Read the model definition and answer for the solid it produces. Units are mm, in the model's axes. A direction names the side the tool comes from. Round coordinates to 2 decimals unless told otherwise and drop trailing zeros. Order: outer loops, then holes, each group sorted by start corner. A loop starts at its lowest first (then second) coordinate and runs counter-clockwise, first axis right, second up. Notation, with made-up numbers: (70.25, 54.25) -> (78.25, 54.25) arc R9 cw to (78.25, 66.25) -> close; hole circle Ø2 at (89, 15). An arc over 180 degrees is marked (long way). One line per item, written item: value. Start each with the question number.
1. Section A-A (z = -1.5) is taken. Give the vertices of the cut face in (x, y).
2. Consider line 1 (Y direction, x = 12, z = 1.05); line 2 (Y direction, x = -12, z = 2.6); line 3 (Y direction, x = 5.5, z = 9.5). Determine where each line is inside the solid, lowest interval first.
3. Section B-B (x = 0) is taken. Give the vertices of the cut face in (y, z) (3 decimals).
4. Section D-D (z = 6.5) is taken. Give the vertices of the cut face in (x, y), then the cut area to 3 significant figures.
5. Section C-C (y = 70.5) is taken. Give the vertices of the cut face in (x, z), then the cut area to 3 significant figures.
6. The mould has two halves that part along Y. Classify faces 4 (the face through (-0.275, 132.886, 12.497)), 5 (the face through (-15.5, 77, 8)), 6 (the face through (0, 2, 9)), 7 (the face through (-12, 147, 3.5)): released by +Y, released by -Y, zero draft, split by the parting line, or undercut.
7. For faces 1 (the face through (0, 63, 8)), 2 (the face through (11.1, 148.5, -1.7)), 3 (the face through (0, 77, 15.5)), determine the directions among +Z, -Z, +X, -X, +Y, -Y from which every point of the face is accessible in a straight line to the end or side of a thin tool.
8. Flat-ended cylindrical pins translate along their axes: pin 1 Ø4 at (x, y) = (9.5, 83.5) entering from -Z; pin 2 Ø1 at (x, y) = (-12.5, 147) entering from -Z. Find the tip coordinate at first contact, or state that the pin passes through.
from build123d import *

# Parameters (mm, degrees)
SKETCH1_R            = 12.5
BOSS_EXTRUDE1_DEPTH  = 150.5
BOSS_EXTRUDE2_DEPTH  = 148.5
SKETCH8_R            = 12.5
CUT_EXTRUDE2_DEPTH   = 152.706130397
BOSS_EXTRUDE7_DEPTH  = 8
BOSS_EXTRUDE8_START  = -121
BOSS_EXTRUDE8_DEPTH  = 121
BOSS_EXTRUDE9_DEPTH  = 148.5
SKETCH13_R           = 1.75
CUT_EXTRUDE3_DEPTH   = 3.5
SKETCH14_R           = 1.75
BOSS_EXTRUDE10_DEPTH = 3.4
SKETCH15_R           = 1.75
CUT_EXTRUDE4_DEPTH   = 3.5
SKETCH16_R           = 1.75
BOSS_EXTRUDE11_DEPTH = 3.4


with BuildPart() as part:
    # Sketch1 → Boss-Extrude1 (new body)
    with BuildSketch(Plane(origin=(0, 0, 0), x_dir=(1, 0, 0), z_dir=(0, 1, 0))):
        with Locations(Location((0, 0, 0), (0, 0, 270))):
            Circle(SKETCH1_R)
    extrude(amount=BOSS_EXTRUDE1_DEPTH)

    # Sketch2 → Boss-Extrude2 (add)
    with BuildSketch(Plane(origin=(0, 150.5, 0), x_dir=(1, 0, 0), z_dir=(0, 1, 0))):
        with BuildLine():
            Line((-13.5, 0), (13.5, 0))
            ThreePointArc((13.5, 0), (0, -13.5), (-13.5, 0))
        make_face()
    extrude(amount=-BOSS_EXTRUDE2_DEPTH)

    # Sketch8 → Cut-Extrude2 (cut, through all)
    with BuildSketch(Plane(origin=(0, 150.5, 0), x_dir=(1, 0, 0), z_dir=(0, 1, 0))):
        Circle(SKETCH8_R)
    extrude(amount=-CUT_EXTRUDE2_DEPTH, mode=Mode.SUBTRACT)

    # Sketch9 → Boss-Extrude7 (add)
    with BuildSketch(Plane(origin=(0, 150.5, 0), x_dir=(1, 0, 0), z_dir=(0, 1, 0))):
        with BuildLine():
            Line((12.5, 0), (1.875, 0))
            ThreePointArc((1.875, 0), (0, -1.875), (-1.875, 0))
            Line((-1.875, 0), (-12.5, 0))
            ThreePointArc((-12.5, 0), (0, -12.5), (12.5, 0))
        make_face()
    extrude(amount=-BOSS_EXTRUDE7_DEPTH)

    # Sketch11 → Boss-Extrude8 (add)
    with BuildSketch(Plane.XZ.offset(-2).offset(BOSS_EXTRUDE8_START)):
        with BuildLine():
            Line((-12.5, 0), (-8, 0))
            ThreePointArc((-8, 0), (0, 8), (8, 0))
            Line((8, 0), (12.5, 0))
            ThreePointArc((12.5, 0), (0, 12.5), (-12.5, 0))
        make_face()
    extrude(amount=BOSS_EXTRUDE8_DEPTH)

    # Sketch12 → Boss-Extrude9 (add)
    with BuildSketch(Plane(origin=(0, 150.5, 0), x_dir=(1, 0, 0), z_dir=(0, 1, 0))):
        with BuildLine():
            Line((-13.5, 0), (-15.5, 0))
            Line((-15.5, 0), (-15.5, -15.5))
            Line((-15.5, -15.5), (15.5, -15.5))
            Line((15.5, -15.5), (15.5, 0))
            Line((15.5, 0), (13.5, 0))
            ThreePointArc((13.5, 0), (0, -13.5), (-13.5, 0))
        make_face()
    extrude(amount=-BOSS_EXTRUDE9_DEPTH)

    # Sketch13 → Cut-Extrude3 (cut)
    with BuildSketch(Plane(origin=(0, 0, 0), x_dir=(-1, 0, 0), z_dir=(0, 0, -1))):
        with Locations((12, 147)):
            Circle(SKETCH13_R)
    extrude(amount=-CUT_EXTRUDE3_DEPTH, mode=Mode.SUBTRACT)

    # Sketch14 → Boss-Extrude10 (add)
    with BuildSketch(Plane(origin=(0, 0, 0), x_dir=(-1, 0, 0), z_dir=(0, 0, -1))):
        with Locations((-12, 147)):
            Circle(SKETCH14_R)
    extrude(amount=BOSS_EXTRUDE10_DEPTH)

    # Sketch15 → Cut-Extrude4 (cut)
    with BuildSketch(Plane(origin=(0, 0, 0), x_dir=(-1, 0, 0), z_dir=(0, 0, -1))):
        with Locations((-12, 5.5)):
            Circle(SKETCH15_R)
    extrude(amount=-CUT_EXTRUDE4_DEPTH, mode=Mode.SUBTRACT)

    # Sketch16 → Boss-Extrude11 (add)
    with BuildSketch(Plane(origin=(0, 0, 0), x_dir=(-1, 0, 0), z_dir=(0, 0, -1))):
        with Locations((12, 5.5)):
            Circle(SKETCH16_R)
    extrude(amount=BOSS_EXTRUDE11_DEPTH)


solid = part.part
Answer:
1. outline: circle Ø3.5 at (-12, 5.5); circle Ø3.5 at (12, 147)
2. line 1: 2 to 3.75, 7.25 to 123, 142.5 to 150.5
2. line 2: 2 to 123, 142.5 to 145.25, 148.75 to 150.5
2. line 3: 2 to 123, 142.5 to 150.5
3. outline: (2, 8) -> (123, 8) -> (123, 12.5) -> (142.5, 12.5) -> (142.5, 1.875) -> (150.5, 1.875) -> (150.5, 15.5) -> (2, 15.5) -> close
4. outline: (-15.5, 2) -> (-4.66, 2) -> (-4.66, 123) -> (-10.68, 123) -> (-10.68, 142.5) -> (10.68, 142.5) -> (10.68, 123) -> (4.66, 123) -> (4.66, 2) -> (15.5, 2) -> (15.5, 150.5) -> (-15.5, 150.5) -> close
4. area: 3,060 mm^2
5. outline: (-15.5, 0) -> (-8, 0) arc R8 cw to (8, 0) -> (15.5, 0) -> (15.5, 15.5) -> (-15.5, 15.5) -> close
5. area: 380 mm^2
6. face 4: undercut
6. face 5: zero draft
6. face 6: released by -Y
6. face 7: undercut
7. face 1: -Z, -Y
7. face 2: -Z
7. face 3: +Z, +X, -X, +Y, -Y
8. pin 1: z = 0
8. pin 2: z = 3.5
